```python
from build123d import *

# Parameters (mm, degrees)
F0_R          = 15
F1_DEPTH      = 5.5
F2_R          = 2
F3_R          = 1
F4_DEPTH      = 15
F6_DEPTH      = 15.001
F6_DEPTH_BACK = 15.001
F8_DEPTH      = 15.001
F8_DEPTH_BACK = 15.001


with BuildPart() as f1:
    # F0 (on Top) → F1 (new body)
    with BuildSketch(Plane.XY):
        Circle(F0_R)
    extrude(amount=F1_DEPTH)

    # F2
    f2_edges = [f1.edges().sort_by_distance(p)[0] for p in [
        (-15, 0, 0),
    ]]
    fillet(f2_edges, radius=F2_R)

    # F3 (on face) → F4 (join)
    with BuildSketch(Plane.XY.offset(5.5)):
        Circle(F3_R)
    extrude(amount=F4_DEPTH)

    # F5 (on Front) → F6 (cut, two sides)
    with BuildSketch(Plane.XZ) as f6_sk:
        Polygon((1, 20.5), (0.125, 20.5), (1, 18), align=None)
        Polygon((-0.125, 20.5), (-1, 20.5), (-1, 18), align=None)
    extrude(amount=-F6_DEPTH, mode=Mode.SUBTRACT)
    extrude(f6_sk.sketch, amount=F6_DEPTH_BACK, mode=Mode.SUBTRACT)

    # F7 (on Right) → F8 (cut, two sides)
    with BuildSketch(Plane.YZ) as f8_sk:
        Polygon((-0.9921567416, 20.5), (-1, 20.5), (-1, 18), (-0.125, 20.5), align=None)
        Polygon((1, 20.5), (0.9921567416, 20.5), (0.125, 20.5), (1, 18), align=None)
    extrude(amount=F8_DEPTH, mode=Mode.SUBTRACT)
    extrude(f8_sk.sketch, amount=-F8_DEPTH_BACK, mode=Mode.SUBTRACT)


solid = f1.part
```
Here's how the part is built. I have some questions about the finished solid (model axes, mm). A direction names the side the tool comes from. Round coordinates to 2 decimals unless told otherwise and drop trailing zeros. Write each loop counter-clockwise with the first axis right and the second up, starting at its lowest first coordinate (ties: lowest second). Pieces come first, ordered by that corner, then holes.
Q1. Please list where these lines run through material, in increasing order: probe 1 along Z at (x, y) = (-1.5, 12); probe 2 along Z at (x, y) = (4.5, 13.75); probe 3 along Y at (x, z) = (0.25, 16).
Q2. Will these pins go through, and if not, where does the flat tip stop? P1, Ø4, axis at x = 6, z = 6, coming from the +Y side; P2, Ø6, axis at x = -8, y = -7, coming from the +Z side; P3, Ø3, axis at y = -1, z = 16.5, coming from the -X side.
Q3. Which directions (+Z, -Z, +X, -X, +Y, -Y) give clear straight access to the entire face, cutting with the end or side of a thin tool? Please do faces 1 (the cylindrical face through (-14.985, 0.66, 3.726)), 2 (the cylindrical face through (0, -1, 12)).
Q4. If we section it at A-A on z = 11.5: Write out the boundary of the cut face in (x, y).
Answer below:
1. probe 1: z = 0 to 5.5
1. probe 2: z = 0.64 to 5.5
1. probe 3: y = -0.97 to 0.97
2. P1: stops at y = 14.44
2. P2: stops at z = 5.5
2. P3: stops at x = -1
3. face 1: +Z, -Z
3. face 2: +Z
4. outline: circle Ø2 at (0, 0)
